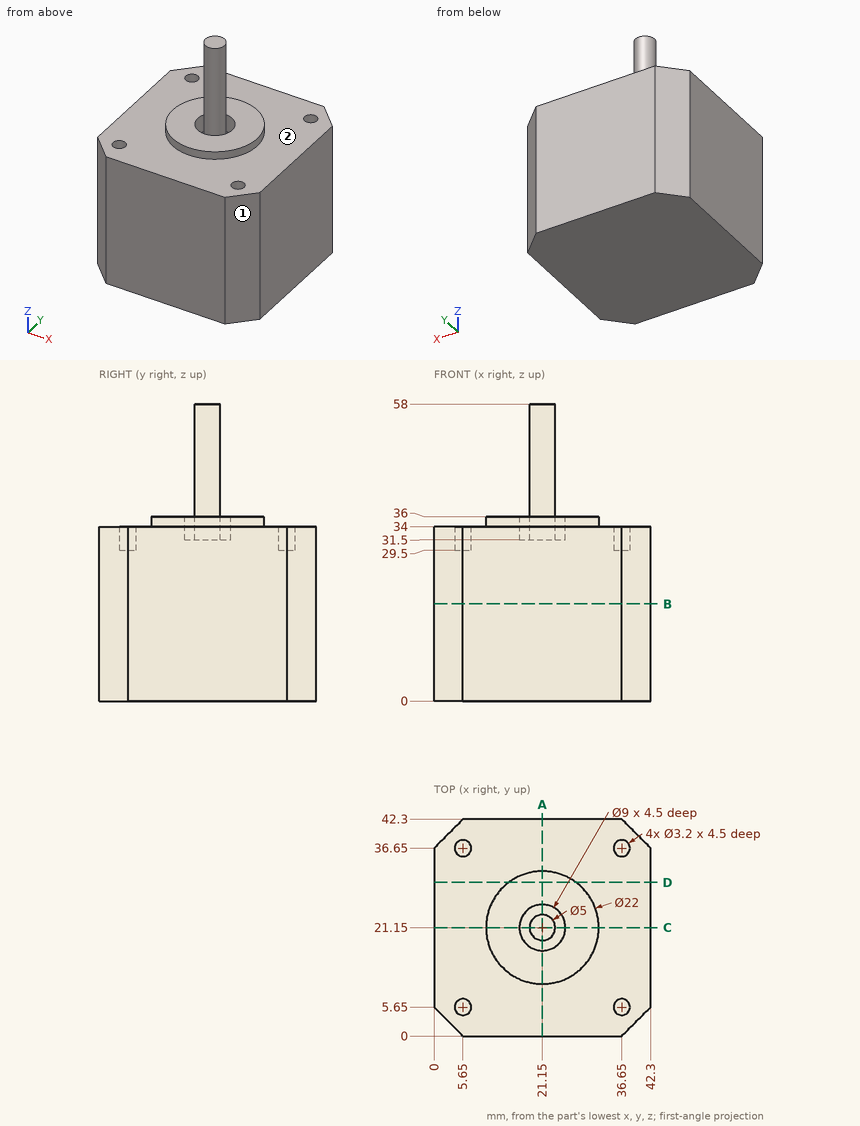
Design review of the part shown in the three views and the two pictorial views. Dimensions are in mm from the part's minimum x, y and z. A direction names the side the tool comes from. Round coordinates to 2 decimals unless told otherwise and drop trailing zeros. Loops run counter-clockwise (first coordinate to the right, second up) from the corner with the lowest first, then second, coordinate; pieces in that order, holes last.
Q1. Insertion check: pin 1 Ø10 at (x, z) = (15.5, 44) entering from -Y; pin 2 Ø3.5 at (x, y) = (36, 6) entering from +Z; pin 3 Ø1 at (x, y) = (36.5, 36.5) entering from +Z. Each pin has a flat end and moves straight along its axis. Give the tip position at first contact, or say it passes through.
Result sheet:
pin 1: stops at y = 18.74
pin 2: stops at z = 34
pin 3: stops at z = 29.5
Q2. Add section D-D on y = 30. Write out the cut boundary in (x, z).
Result sheet:
outline: (0, 0) - (42.3, 0) - (42.3, 34) - (27.68, 34) - (27.68, 36) - (14.62, 36) - (14.62, 34) - (0, 34) - close
Q3. Add section B-B on z = 19. Write out the cut boundary in (x, y), plus the area to 3 significant figures.
Result sheet:
outline: (0, 5.65) - (5.65, 0) - (36.65, 0) - (42.3, 5.65) - (42.3, 36.65) - (36.65, 42.3) - (5.65, 42.3) - (0, 36.65) - close
area: 1,730 mm2
Q4. Machinability: for the marked faces 1 and 2, which of the approach directions +Z, -Z, +X, -X, +Y, -Y give a long, thin tool a straight path to every point of the face, cutting with its end or side? Answer none if there is none.
Result sheet:
face 1: +Z, -Z, +X, -Y
face 2: +Z
Q5. Add section A-A on x = 21.15. Write out the cut boundary in (y, z), plus the area to 3 significant figures.
Result sheet:
outline: (0, 0) - (42.3, 0) - (42.3, 34) - (32.15, 34) - (32.15, 36) - (25.65, 36) - (25.65, 31.5) - (23.65, 31.5) - (23.65, 58) - (18.65, 58) - (18.65, 31.5) - (16.65, 31.5) - (16.65, 36) - (10.15, 36) - (10.15, 34) - (0, 34) - close
area: 1,570 mm2
Q6. To check wall thickness, follow line 1 along Y through (x, z) = (36.65, 31.75); line 2 along Y through (x, z) = (21, 32). State the ranges of each line that lie inside material, in increasing order.
Result sheet:
line 1: y = 0 to 4.05, 7.25 to 35.05, 38.25 to 42.3
line 2: y = 0 to 16.65, 18.65 to 23.65, 25.65 to 42.3
